Autodesk Inventor part; units mm, degrees
ref_plane "YZ Plane" through (0, 0, 0) normal (1, 0, 0) x (0, 1, 0)
ref_plane "XZ Plane" through (0, 0, 0) normal (0, 1, 0) x (-1, 0, 0)
ref_plane "XY Plane" through (0, 0, 0) normal (0, 0, 1) x (1, 0, 0)
sketch "Sketch1" plane through (0, 0, 0) normal (0, 1, 0) x (-1, 0, 0)
  line L0 (-18, 25) -> (18, 25)
  line L1 (25, 18) -> (25, -18)
  line L2 (18, -25) -> (-18, -25)
  line L3 (-25, -18) -> (-25, 18)
  line L4 (-25, 25) -> (25, -25) construction
  line L5 (25, 25) -> (-25, -25) construction
  circle A0 centre (0, 0) radius 2.75
  arc A1 (25, 18) -> (18, 25) centre (18, 18) ccw
  arc A2 (18, -25) -> (25, -18) centre (18, -18) ccw
  arc A3 (-25, -18) -> (-18, -25) centre (-18, -18) ccw
  arc A4 (-18, 25) -> (-25, 18) centre (-18, 18) ccw
  line L6 (-20.2, 20.2) -> (20.2, 20.2)
  line L7 (20.2, 20.2) -> (20.2, -20.2)
  line L8 (20.2, -20.2) -> (-20.2, -20.2)
  line L9 (-20.2, -20.2) -> (-20.2, 20.2)
  line L10 (-20.2, 20.2) -> (20.2, -20.2) construction
  line L11 (20.2, 20.2) -> (-20.2, -20.2) construction
  line L12 (20.6, -20.6) -> (20.6, 20.6)
  line L13 (20.6, 20.6) -> (-20.6, 20.6)
  line L14 (-20.6, 20.6) -> (-20.6, -20.6)
  line L15 (-20.6, -20.6) -> (20.6, -20.6)
  dimension "d0" = 50
  dimension "d1" = 50
  dimension "d2" = 5.5
  dimension "d3" = 7
  dimension "d4" = 40.4
  dimension "d5" = 40.4
  dimension "d8" = 0.4
extrude "Extrusion1" add sketch "Sketch1" against normal blind 35 contours L0 A1 L1 A2 L2 A3 L3 A4 | A0 | L6 L7 L8 L9 | L15 L14 L13 L12
fillet "Fillet1" radius 5 8 edges at (0, -35, 25) (-22.9497, -35, 22.9497) (-25, -35, 0) (-22.9497, -35, -22.9497) (0, -35, -25) (22.9497, -35, -22.9497) (25, -35, 0) (22.9497, -35, 22.9497)
extrude "Extrusion2" cut sketch "Sketch1" against normal blind 25 contours A0 | L6 L7 L8 L9 | L15 L14 L13 L12
sketch "Sketch2" plane through (0, -35, 0) normal (0, -1, 0) x (1, 0, 0)
  circle A0 centre (0, 0) radius 2.75
  line L0 (-10.5, 12.5) -> (10.5, 12.5)
  arc A1 (-10.5, 12.5) -> (-12.5, 10.5) centre (-10.5, 10.5) ccw
  line L1 (-12.5, -10.5) -> (-12.5, 10.5)
  arc A2 (-12.5, -10.5) -> (-10.5, -12.5) centre (-10.5, -10.5) ccw
  line L2 (10.5, -12.5) -> (-10.5, -12.5)
  arc A3 (10.5, -12.5) -> (12.5, -10.5) centre (10.5, -10.5) ccw
  line L3 (12.5, 10.5) -> (12.5, -10.5)
  arc A4 (12.5, 10.5) -> (10.5, 12.5) centre (10.5, 10.5) ccw
  circle A5 centre (0, 0) radius 5
  dimension "d12" = 10
properties part number "PATA_PLASTICO" material "Steel, Mild, Welded"
Geometry: final body of the model. Coordinates: model frame, mm. A direction names the side the tool comes from. Round coordinates to 2 decimals unless told otherwise and drop trailing zeros. Order: outer loops, then holes, each group sorted by start corner. A loop starts at its lowest first (then second) coordinate and runs counter-clockwise, first axis right, second up. Notation, with made-up numbers: (53.5, 38) - (60.5, 38) arc R11 ccw to (60.5, 53) - close; hole circle Ø3 at (53.5, -37). An arc over 180 degrees is marked (long way). Use CSV: the item, a comma, the result in double quotes. Start each with the question number.
Q1. First-contact query: pin 1 (6 mm diameter, centred on x = -2, z = -3.5, fed in from +Y). Flat tip, straight axial feed; report the tip coordinate or a pass-through.
Q2. Access query for faces 1 (the face through (0, -35, 0)), 2 (the face through (0, -12, 20.6)). Directions: +Z, -Z, +X, -X, +Y, -Y. A direction counts if a zero-diameter tool reaches every point of the face in a straight line with its end or side. Return the directions, or none.
Q3. Section query D-D (y = -29). Return loops of the section in (x, z).
Q4. Mould query, pull axis X, two halves, no side actions, for faces 3 (the face through (23, -14.8, -22.9)), 4 (the face through (20.6, -12, 0)), 5 (the face through (0, -15, -25)). Classes: +X half, -X half, draft (parallel to the pull), parting line (faces both ways), or undercut.
Q5. Section query A-A (y = -10). Return loops of the section in (x, z), and give its area (4 significant figures).
Q6. Section query B-B (x = 5). Return loops of the section in (y, z), and give its area (3 significant figures).
Q7. Section query C-C (z = -9.5). Return loops of the section in (x, y), and give its area (3 significant figures).
Q8. Material intervals for line 1 along Z through (x, y) = (15, -17); line 2 along Y through (x, z) = (4, 9.5), sorted ascending. Write a range as from..to.
Result set:
1,pin 1,"stops at y = -25"
2,face 1,"+Z, -Z, +X, -X, -Y"
2,face 2,"+Y"
3,outline,"(-25, -18) arc R7 ccw to (-18, -25) - (18, -25) arc R7 ccw to (25, -18) - (25, 18) arc R7 ccw to (18, 25) - (-18, 25) arc R7 ccw to (-25, 18) - close"
4,face 3,"+X half"
4,face 4,"undercut"
4,face 5,"draft"
5,outline,"(-25, -18) arc R7 ccw to (-18, -25) - (18, -25) arc R7 ccw to (25, -18) - (25, 18) arc R7 ccw to (18, 25) - (-18, 25) arc R7 ccw to (-25, 18) - close; hole (-20.6, -20.6) - (20.6, -20.6) - (20.6, 20.6) - (-20.6, 20.6) - close"
5,area,"760.5 mm2"
6,outline,"(-35, -20) arc R5 ccw to (-30, -25) - (0, -25) - (0, -20.6) - (-25, -20.6) - (-25, 20.6) - (0, 20.6) - (0, 25) - (-30, 25) arc R5 ccw to (-35, 20) - close"
6,area,"709 mm2"
7,outline,"(-25, -30) arc R5 ccw to (-20, -35) - (20, -35) arc R5 ccw to (25, -30) - (25, 0) - (20.6, 0) - (20.6, -25) - (-20.6, -25) - (-20.6, 0) - (-25, 0) - close"
7,area,"709 mm2"
8,line 1,"z = -25..-20.6, 20.6..25"
8,line 2,"y = -35..-25"
